Can you work these out from the drawing? Everything is in mm from the part's minimum corner. A direction names the side the tool comes from. Round coordinates to 2 decimals unless told otherwise and drop trailing zeros. Loops run counter-clockwise (first coordinate to the right, second up) from the corner with the lowest first, then second, coordinate; pieces in that order, holes last. Notation, with made-up numbers: (-34, 79.5) -> (16, 79.5) arc R23 cw to (16, 116.5) -> close; hole circle Ø9 at (-2, 48.5). An arc over 180 degrees is marked (long way). Answer as a JSON object with one key per item and string values.
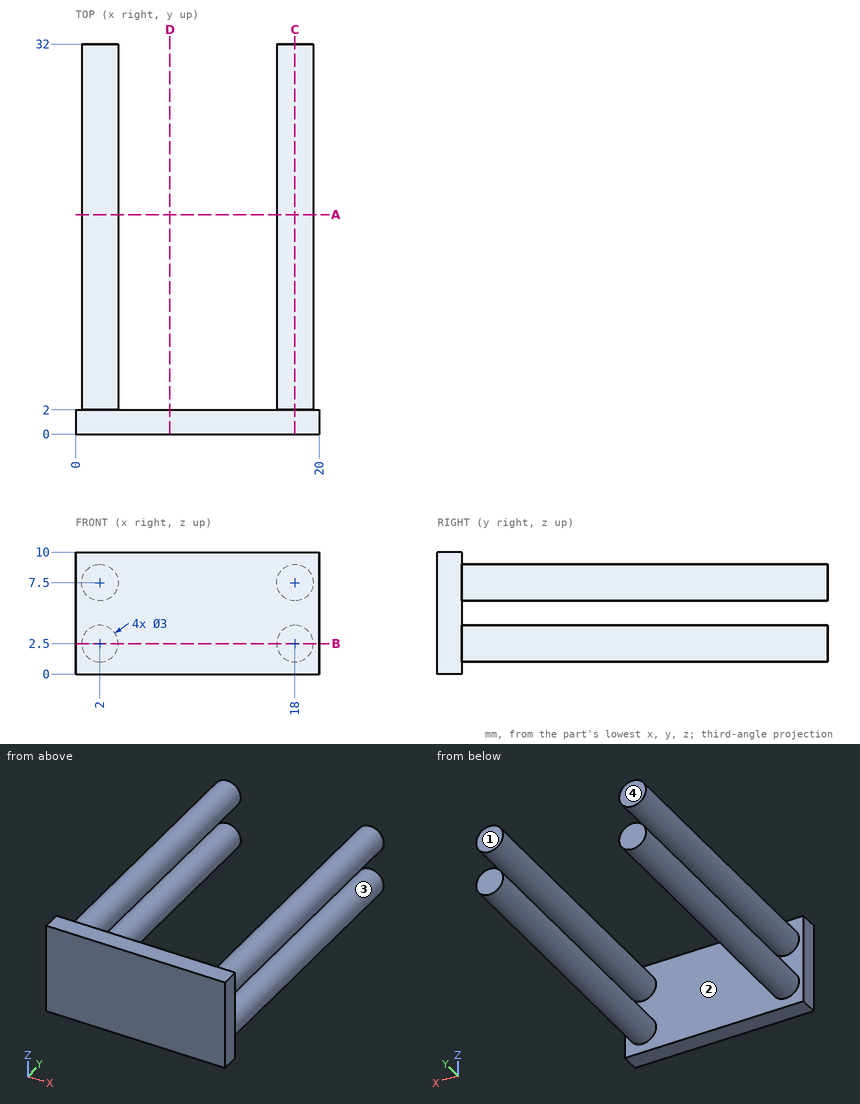
Q1. On a 3-axis mill with a long thin cutter (end or side, diameter ignored), from which of +Z, -Z, +X, -X, +Y, -Y can I reach the whole of each face in a straight line? I mean the marked faces 1 and 2. Say none if no direction works.
Determined:
{"face 1": "+Z, -Z, +X, -X, +Y", "face 2": "+Y"}
Q2. I want a section at C-C, the plane x = 18. Write out the boundary of the cut face in (y, z).
Determined:
{"outline": "(0, 0) -> (2, 0) -> (2, 1) -> (32, 1) -> (32, 4) -> (2, 4) -> (2, 6) -> (32, 6) -> (32, 9) -> (2, 9) -> (2, 10) -> (0, 10) -> close"}
Q3. We'd pull the mould along Z, two halves only. Please class the marked faces 3 and 4: pulls with the +Z half, pulls with the -Z half, needs draft (parallel to the pull), parting line crosses it, or undercut.
Determined:
{"face 3": "undercut", "face 4": "needs draft"}
Q4. I want a section at B-B, the plane z = 2.5. Write out the boundary of the cut face in (x, y), then the cut area to 3 significant figures.
Determined:
{"outline": "(0, 0) -> (20, 0) -> (20, 2) -> (19.5, 2) -> (19.5, 32) -> (16.5, 32) -> (16.5, 2) -> (3.5, 2) -> (3.5, 32) -> (0.5, 32) -> (0.5, 2) -> (0, 2) -> close", "area": "220 mm²"}
Q5. I want a section at A-A, the plane y = 18. Write out the boundary of the cut face in (x, z), then the cut area to 3 significant figures.
Determined:
{"outline": "circle Ø3 at (2, 2.5); circle Ø3 at (2, 7.5); circle Ø3 at (18, 2.5); circle Ø3 at (18, 7.5)", "area": "28.3 mm²"}
Q6. I'm going to push a flat-ended pin straight in: pin 1 (5 mm diameter, centred on x = 11.5, z = 3.5, fed in from +Y). Where does the tip first touch, or does it pass through?
Determined:
{"pin 1": "y = 2"}
Q7. I want a section at D-D, the plane x = 7.75. Write out the boundary of the cut face in (y, z).
Determined:
{"outline": "(0, 0) -> (2, 0) -> (2, 10) -> (0, 10) -> close"}
Q8. If I drill on L1, parallel to Y at x = 5, z = 5; L2, parallel to X at y = 25, z = 3.75; L3, parallel to X at y = 20.5, z = 7.75, over which ranges is the centre line in solid material (lowest first)? Write a range as [from, to].
Determined:
{"L1": "[0, 2]", "L2": "[1.17, 2.83], [17.17, 18.83]", "L3": "[0.52, 3.48], [16.52, 19.48]"}
